Read the model definition and answer for the solid it produces. Units are mm, in the model's axes. Give positions to 0.01 mm unless a question says otherwise; leave off trailing zeros. Loops run counter-clockwise (first coordinate to the right, second up) from the corner with the lowest first, then second, coordinate; pieces in that order, holes last.
(1) Find section C-C, the plane y = 2.6. Write down the section's boundary in (x, z) (3 decimals), then the cut area to 3 significant figures.
(2) Determine the mould class of faces 1 (the face through (-55, 0, 55)), 2 (the face through (-123.98, 2.63, -27.53)), 3 (the face through (53.92, 2.63, 81.84)) for opening direction Z: pulls with the +Z half, pulls with the -Z half, needs draft (parallel to the pull), parting line crosses it, or undercut.
(3) Straight lines are drawn through the part: probe 1 along X at (y, z) = (3.2, -78.74) (3 decimals); probe 2 along X at (y, z) = (0.4, -78); probe 3 along Z at (x, y) = (54.61, 1.65) (3 decimals). For each, find the intervals that lie inside material, in ascending order.
(4) Find section A-A, the plane x = 0. Write down the section's boundary in (y, z), then the cut area to 3 significant figures.
(5) This flat-tipped pin is pushed along its axis until it touches: P1, Ø3, axis at x = 18.5, y = 4.5, coming from the +Z side. Where does it stop, or does it pass through?
(6) Find section B-B, the plane z = 0. Write down the section's boundary in (x, y).
(7) Find section D-D, the plane x = 54.61. Write down the section's boundary in (y, z) (3 decimals), then the cut area to 3 significant figures.
```python
from build123d import *

# Parameters (mm, degrees)
SKETCH1_R          = 127
BASE_DEPTH         = 5.334
SKETCH2_R          = 76.2
CUT_EXTRUDE1_DEPTH = 180.684310823
HOLE2_OUTLINE_R    = 3.175
HOLE2_DEPTH        = 5.334


# Read off the part's stored shape, not the designer's step: Hole2
with BuildPart() as part:
    # Sketch1 → Base (new body)
    with BuildSketch(Plane(origin=(0, 0, 0), x_dir=(1, 0, 0), z_dir=(0, 1, 0))):
        with Locations(Location((0, 0, 0), (0, 0, 270))):
            Circle(SKETCH1_R)
    extrude(amount=BASE_DEPTH)

    # Sketch2 → Cut-Extrude1 (cut, through all)
    with BuildSketch(Plane(origin=(0, 5.334, 0), x_dir=(1, 0, 0), z_dir=(0, 1, 0))):
        with Locations(Location((0, 0, 0), (0, 0, 270))):
            Circle(SKETCH2_R)
    extrude(amount=-CUT_EXTRUDE1_DEPTH, mode=Mode.SUBTRACT)

    # Hole2 outline → Hole2 (cut)
    with BuildSketch(Plane(origin=(0, 0, 0), x_dir=(1, 0, 0), z_dir=(0, 1, 0))):
        with Locations((-54.61, -78.74)):
            Circle(HOLE2_OUTLINE_R)
        with Locations((54.61, -78.74)):
            Circle(HOLE2_OUTLINE_R)
        with Locations((54.61, 78.74)):
            Circle(HOLE2_OUTLINE_R)
        with Locations((-54.61, 78.74)):
            Circle(HOLE2_OUTLINE_R)
    extrude(amount=HOLE2_DEPTH, mode=Mode.SUBTRACT)


solid = part.part
```
Entries:
1. outline: circle Ø254 at (0, 0); hole circle Ø152.4 at (0, 0); hole circle Ø6.35 at (-54.61, -78.74); hole circle Ø6.35 at (-54.61, 78.74); hole circle Ø6.35 at (54.61, -78.74); hole circle Ø6.35 at (54.61, 78.74)
1. area: 32,300 mm2
2. face 1: needs draft
2. face 2: parting line crosses it
2. face 3: undercut
3. probe 1: x = -99.644 to -57.785, -51.435 to 51.435, 57.785 to 99.644
3. probe 2: x = -100.22 to -57.7, -51.52 to 51.52, 57.7 to 100.22
3. probe 3: z = -114.659 to -81.915, -75.565 to -53.143, 53.143 to 75.565, 81.915 to 114.659
4. outline: (0, -127) - (5.33, -127) - (5.33, -76.2) - (0, -76.2) - close; (0, 76.2) - (5.33, 76.2) - (5.33, 127) - (0, 127) - close
4. area: 542 mm2
5. P1: stops at z = 125.86
6. outline: (-127, 0) - (-76.2, 0) - (-76.2, 5.33) - (-127, 5.33) - close; (76.2, 0) - (127, 0) - (127, 5.33) - (76.2, 5.33) - close
7. outline: (0, -114.659) - (5.334, -114.659) - (5.334, -81.915) - (0, -81.915) - close; (0, -75.565) - (5.334, -75.565) - (5.334, -53.143) - (0, -53.143) - close; (0, 53.143) - (5.334, 53.143) - (5.334, 75.565) - (0, 75.565) - close; (0, 81.915) - (5.334, 81.915) - (5.334, 114.659) - (0, 114.659) - close
7. area: 589 mm2
